Source: three-view drawing plus pictorial views. Frame: mm from the lowest corner of the part. A direction names the side the tool comes from. Coordinates: 2 decimals unless noted, no trailing zeros. Write each loop counter-clockwise with the first axis right and the second up, starting at its lowest first coordinate (ties: lowest second). Pieces come first, ordered by that corner, then holes. Notation, with made-up numbers: (-6.75, 44.5) -> (2.25, 44.5) arc R29 cw to (2.25, 70.5) -> close; hole circle Ø9 at (77.25, 36.5). An arc over 180 degrees is marked (long way). One line per item, written item: value. Start each with the question number.
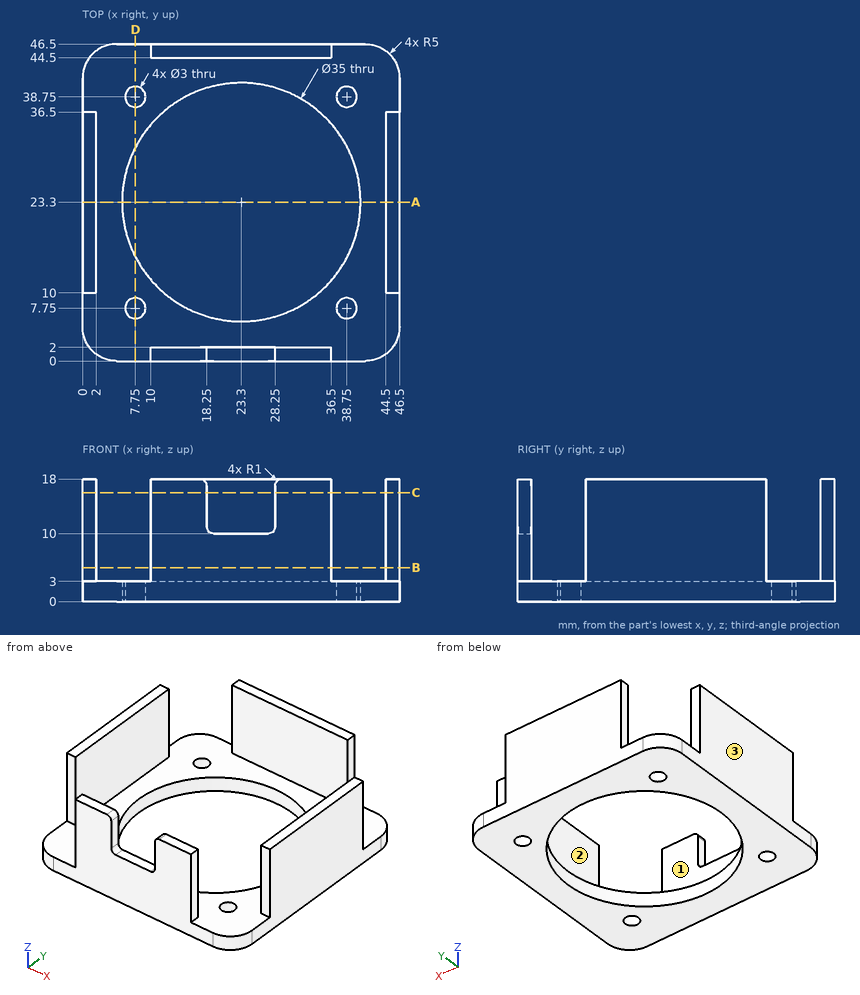
Q1. First-contact query: P1, Ø0.6, axis at y = 45.5, z = 11.5, coming from the +X side; P2, Ø1.6, axis at x = 45.5, z = 13.5, coming from the +Y side; P3, Ø2, axis at y = 45.5, z = 10, coming from the -X side. Flat tips, straight axial feed; report the tip coordinate or a pass-through.
Q2. Cut plane B-B on z = 5. Output: boundary loops of the cut face in (x, y), and give its area (3 significant figures).
Q3. Access query for the marked faces 1, 2 and 3. Directions: +Z, -Z, +X, -X, +Y, -Y. A direction counts if a zero-diameter tool reaches every point of the face in a straight line with its end or side. Return the directions, or none.
Q4. Line query: L1, parallel to X at y = 32, z = 9.5; L2, parallel to Y at x = 38.75, z = 1.9. Output: solid intervals per line, ascending. Write a range as from..to.
Q5. Cut plane A-A on y = 23.3. Output: boundary loops of the cut face in (x, z).
Q6. Cut plane C-C on z = 16. Output: boundary loops of the cut face in (x, y).
Q7. Cut plane D-D on x = 7.75. Output: boundary loops of the cut face in (y, z).
Solution:
1. P1: x = 36.5
1. P2: y = 36.5
1. P3: x = 10
2. outline: (0, 10) -> (2, 10) -> (2, 36.5) -> (0, 36.5) -> close; (10, 0) -> (36.5, 0) -> (36.5, 2) -> (10, 2) -> close; (10, 44.5) -> (36.5, 44.5) -> (36.5, 46.5) -> (10, 46.5) -> close; (44.5, 10) -> (46.5, 10) -> (46.5, 36.5) -> (44.5, 36.5) -> close
2. area: 212 mm²
3. face 1: +Z, +X, -X
3. face 2: +Z, +Y, -Y
3. face 3: +Z, -Z, -X, +Y, -Y
4. L1: 0..2, 44.5..46.5
4. L2: 0..6.25, 9.25..15.08, 31.52..37.25, 40.25..46.5
5. outline: (0, 0) -> (5.8, 0) -> (5.8, 3) -> (2, 3) -> (2, 18) -> (0, 18) -> close; (40.8, 0) -> (46.5, 0) -> (46.5, 18) -> (44.5, 18) -> (44.5, 3) -> (40.8, 3) -> close
6. outline: (0, 10) -> (2, 10) -> (2, 36.5) -> (0, 36.5) -> close; (10, 0) -> (18.25, 0) -> (18.25, 2) -> (10, 2) -> close; (10, 44.5) -> (36.5, 44.5) -> (36.5, 46.5) -> (10, 46.5) -> close; (28.25, 0) -> (36.5, 0) -> (36.5, 2) -> (28.25, 2) -> close; (44.5, 10) -> (46.5, 10) -> (46.5, 36.5) -> (44.5, 36.5) -> close
7. outline: (0, 0) -> (6.25, 0) -> (6.25, 3) -> (0, 3) -> close; (9.25, 0) -> (15.27, 0) -> (15.27, 3) -> (9.25, 3) -> close; (31.33, 0) -> (37.25, 0) -> (37.25, 3) -> (31.33, 3) -> close; (40.25, 0) -> (46.5, 0) -> (46.5, 3) -> (40.25, 3) -> close
